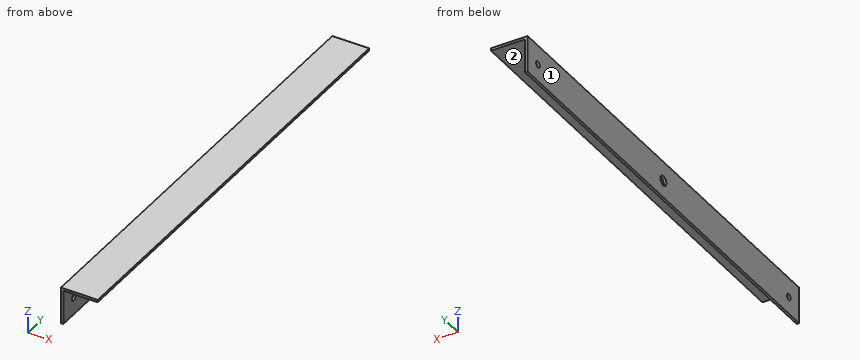
from build123d import *

# Parameters (mm, degrees)
SKETCH_1_W          = 15
SKETCH_1_H          = 1
EXTRUDE_1_DEPTH     = 184
SKETCH_3_W          = 1
SKETCH_3_H          = 184
EXTRUDE_2_DEPTH     = 14
M3X0_5_1_D          = 2.5
SKETCH_7_R          = 2
CUT_EXTRUDE_1_DEPTH = 92


with BuildPart() as part:
    # ｽｹｯﾁ1 → ﾎﾞｽ - 押し出し1 (new body)
    with BuildSketch(Plane(origin=(0, 0, 0), x_dir=(1, 0, 0), z_dir=(0, 1, 0))):
        with Locations((7.5, -0.5)):
            Rectangle(SKETCH_1_W, SKETCH_1_H)
    extrude(amount=EXTRUDE_1_DEPTH)

    # ｽｹｯﾁ3 → ﾎﾞｽ - 押し出し2 (add)
    with BuildSketch(Plane(origin=(0, 0, 0), x_dir=(-1, 0, 0), z_dir=(0, 0, -1))):
        with Locations((-0.5, 92)):
            Rectangle(SKETCH_3_W, SKETCH_3_H)
    extrude(amount=EXTRUDE_2_DEPTH)

    # M3x0.5 ねじ穴1 (through all)
    with Locations(Plane.ZY):
        with Locations((-7, 7), (-7, 177)):
            Hole(M3X0_5_1_D / 2)

    # ｽｹｯﾁ7 → ｶｯﾄ - 押し出し1 (cut)
    with BuildSketch(Plane.ZY):
        with Locations((-7, 92)):
            Circle(SKETCH_7_R)
    extrude(amount=-CUT_EXTRUDE_1_DEPTH, mode=Mode.SUBTRACT)


solid = part.part
The listing builds one solid part. Answer for the finished solid, in the listing's coordinates (mm). Face numbers are marked on the shaded views. A direction names the side the tool comes from. Round coordinates to 2 decimals unless told otherwise and drop trailing zeros. Write each loop counter-clockwise with the first axis right and the second up, starting at its lowest first coordinate (ties: lowest second). Pieces come first, ordered by that corner, then holes. Notation, with made-up numbers: (-8.5, 13.25) - (19.5, 13.25) arc R16 cw to (19.5, 30.25) - close; hole circle Ø3 at (-19.75, -26). An arc over 180 degrees is marked (long way). Use a Markdown table: item, result. Add a question column.
1. The part is cut by section D-D (z = -12.5). Write down the section's boundary in (x, y), and give its area (3 significant figures).
2. Consider line 1 (Y direction, x = 0.6, z = -7); line 2 (Z direction, x = 8, y = 33). Determine where each line is inside the solid, lowest interval first.
3. The part is cut by section A-A (y = 92). Write down the section's boundary in (x, z).
4. The part is cut by section C-C (x = 8.5). Write down the section's boundary in (y, z), and give its area (3 significant figures).
5. The part is cut by section B-B (y = 155.5). Write down the section's boundary in (x, z).
6. Flat-ended cylindrical pins translate along their axes: P1, Ø4.5, axis at y = 92, z = -7, coming from the +X side; P2, Ø1.5, axis at x = 4, y = 148.5, coming from the -Z side; P3, Ø8, axis at x = 3.5, y = 78, coming from the -Z side. Find the tip coordinate at first contact, or state that the pin passes through.
7. A tool of negligible diameter and unlimited length cuts with its end or side. For the marked faces 1 and 2, from which of +Z, -Z, +X, -X, +Y, -Y can it reach the whole face along a straight path? Write none if from no direction.
Reported:
| question | item | result |
|---|---|---|
| 1 | outline | (0, 0) - (1, 0) - (1, 184) - (0, 184) - close |
| 1 | area | 184 mm^2 |
| 2 | line 1 | 0 to 5.75, 8.25 to 90, 94 to 175.75, 178.25 to 184 |
| 2 | line 2 | 0 to 1 |
| 3 | outline | (0, -14) - (1, -14) - (1, -9) - (0, -9) - close; (0, -5) - (1, -5) - (1, 0) - (15, 0) - (15, 1) - (0, 1) - close |
| 4 | outline | (0, 0) - (184, 0) - (184, 1) - (0, 1) - close |
| 4 | area | 184 mm^2 |
| 5 | outline | (0, -14) - (1, -14) - (1, 0) - (15, 0) - (15, 1) - (0, 1) - close |
| 6 | P1 | x = 1 |
| 6 | P2 | z = 0 |
| 6 | P3 | z = -14 |
| 7 | face 1 | +Z, -Z, -X, +Y, -Y |
| 7 | face 2 | -Z, +X, +Y, -Y |
